from build123d import *

# Parameters (mm, degrees)
SKETCH1_W             = 105
SKETCH1_H             = 70
BOSS_EXTRUDE1_DEPTH   = 2.5
F_6_0MM_DOWEL_HOLE1_D = 6


with BuildPart() as part:
    # Sketch1 → Boss-Extrude1 (new body, symmetric)
    with BuildSketch(Plane.XY):
        Rectangle(SKETCH1_W, SKETCH1_H)
    extrude(amount=BOSS_EXTRUDE1_DEPTH, both=True)

    # Ø6.0mm Dowel Hole1 (through all)
    with Locations(Plane.XY.offset(2.5)):
        with Locations((-46.5, 23), (-46.5, -23), (46.5, -23), (46.5, 23)):
            Hole(F_6_0MM_DOWEL_HOLE1_D / 2)


solid = part.part
Part model, mm, in its own coordinate system. Coordinates: 2 decimals unless noted, no trailing zeros. Write each loop counter-clockwise with the first axis right and the second up, starting at its lowest first coordinate (ties: lowest second). Pieces come first, ordered by that corner, then holes. Notation, with made-up numbers: (40, -25.75) - (87, -25.75) arc R19 ccw to (87, -8.75) - close; hole circle Ø4 at (-8.75, 67.5). An arc over 180 degrees is marked (long way). Put each result on its own line as item: value.
1. Two-plate mould, pull along Y, no slides. Class faces 1 (the flat face through (-1, 35, 0)), 2 (the flat face through (-52.5, 0, 0)), 3 (the cylindrical face through (-43.5, -22.9, 0)), 4 (the flat face through (-1, -35, 0)): +Y half, -Y half, draft (parallel to the pull), parting line (faces both ways), or undercut.
Final values:
face 1: +Y half
face 2: draft
face 3: undercut
face 4: -Y half
2. Band-saw the part on B-B (z = -0.4). Write the cut outline in (x, y).
Final values:
outline: (-52.5, -35) - (52.5, -35) - (52.5, 35) - (-52.5, 35) - close; hole circle Ø6 at (-46.5, -23); hole circle Ø6 at (-46.5, 23); hole circle Ø6 at (46.5, -23); hole circle Ø6 at (46.5, 23)
3. Probe line 1 along Y through (x, z) = (-46.5, 0.7); line 2 along Y through (x, z) = (45, 1.5); line 3 along X through (y, z) = (-21.5, -1.6). List the from-to ranges inside material, lowest first. Write a range as [from, to].
Final values:
line 1: y = [-35, -26], [-20, 20], [26, 35]
line 2: y = [-35, -25.6], [-20.4, 20.4], [25.6, 35]
line 3: x = [-52.5, -49.1], [-43.9, 43.9], [49.1, 52.5]
4. Band-saw the part on C-C (x = -46.5). Write the cut outline in (y, z).
Final values:
outline: (-35, -2.5) - (-26, -2.5) - (-26, 2.5) - (-35, 2.5) - close; (-20, -2.5) - (20, -2.5) - (20, 2.5) - (-20, 2.5) - close; (26, -2.5) - (35, -2.5) - (35, 2.5) - (26, 2.5) - close
5. Band-saw the part on A-A (y = 23). Write the cut outline in (x, z), then the cut area to 3 significant figures.
Final values:
outline: (-52.5, -2.5) - (-49.5, -2.5) - (-49.5, 2.5) - (-52.5, 2.5) - close; (-43.5, -2.5) - (43.5, -2.5) - (43.5, 2.5) - (-43.5, 2.5) - close; (49.5, -2.5) - (52.5, -2.5) - (52.5, 2.5) - (49.5, 2.5) - close
area: 465 mm²
6. Flat gauge pin, fed straight in: pin 1 Ø3.5 at (x, y) = (46.5, -23) entering from +Z (3 decimals). Where does the tip first touch, or does it go through?
Final values:
pin 1: passes through
